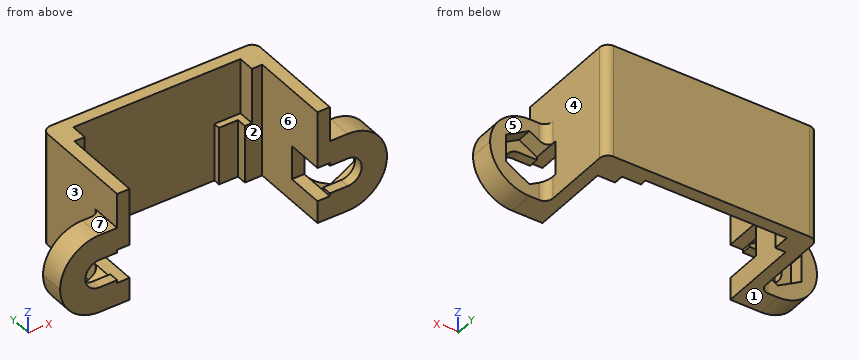
from build123d import *

# Parameters (mm, degrees)
BOSS_EXTRUDE1_DEPTH = 13.7
SKETCH3_W           = 6.9
SKETCH3_H           = 3
BOSS_EXTRUDE2_DEPTH = 9.5
SKETCH4_W           = 1.25
SKETCH4_H           = 2
BOSS_EXTRUDE3_DEPTH = 13.7
BOSS_EXTRUDE4_DEPTH = 7
CUT_EXTRUDE1_DEPTH  = 37.803396582
SKETCH7_W           = 2.15
SKETCH7_H           = 3.4
CUT_EXTRUDE2_DEPTH  = 37.803396582
CUT_EXTRUDE3_DEPTH  = 1.8
CUT_EXTRUDE4_REACH  = 38.457
SKETCH9_W           = 4.099186912
SKETCH9_H           = 4.5
FILLET1_R           = 1
FILLET2_R           = 1


with BuildPart() as part:
    # Sketch2 → Boss-Extrude1 (new body)
    with BuildSketch(Plane.XY):
        Polygon((0, 13.2), (0, 0), (1.5, 0), (1.5, 11.7), (24.2, 11.7), (24.2, 0), (25.7, 0), (25.7, 13.2), align=None)
    extrude(amount=BOSS_EXTRUDE1_DEPTH)

    # Sketch3 → Boss-Extrude2 (add)
    with BuildSketch(Plane(origin=(0, 0, 0), x_dir=(-1, 0, 0), z_dir=(0, 0, -1))):
        with Locations((-29.15, 1.5)):
            Rectangle(SKETCH3_W, SKETCH3_H)
        with Locations((3.45, 1.5)):
            Rectangle(SKETCH3_W, SKETCH3_H)
    extrude(amount=-BOSS_EXTRUDE2_DEPTH)

    # Sketch4 → Boss-Extrude3 (add)
    with BuildSketch(Plane(origin=(0, 0, 0), x_dir=(-1, 0, 0), z_dir=(0, 0, -1))):
        with Locations((-23.575, 10.7)):
            Rectangle(SKETCH4_W, SKETCH4_H)
        with Locations((-2.125, 10.7)):
            Rectangle(SKETCH4_W, SKETCH4_H)
    extrude(amount=-BOSS_EXTRUDE3_DEPTH)

    # Sketch5 → Boss-Extrude4 (add)
    with BuildSketch(Plane(origin=(0, 0, 0), x_dir=(-1, 0, 0), z_dir=(0, 0, -1))):
        Polygon((-22.95, 11.7), (-22.95, 9.7), (-22.1, 9.7), (-22.1, 10.9), (-19.8, 10.9), (-19.8, 11.7), align=None)
    extrude(amount=-BOSS_EXTRUDE4_DEPTH)

    # Sketch6 → Cut-Extrude1 (cut, through all)
    with BuildSketch(Plane(origin=(0, 3, 0), x_dir=(1, 0, 0), z_dir=(0, 1, 0))):
        with BuildLine():
            Line((32.6, -9.5), (32.6, -4.75))
            ThreePointArc((32.6, -4.75), (31.208757211, -8.108757211), (27.85, -9.5))
            Line((27.85, -9.5), (32.6, -9.5))
        make_face()
        with BuildLine():
            Line((32.6, -4.75), (32.6, 0))
            Line((32.6, 0), (27.85, 0))
            ThreePointArc((27.85, 0), (31.208757211, -1.391242789), (32.6, -4.75))
        make_face()
        with BuildLine():
            Line((-2.15, 0), (-6.9, 0))
            Line((-6.9, 0), (-6.9, -4.75))
            ThreePointArc((-6.9, -4.75), (-5.508757211, -1.391242789), (-2.15, 0))
        make_face()
        with BuildLine():
            ThreePointArc((-2.15, -9.5), (-5.508757211, -8.108757211), (-6.9, -4.75))
            Line((-6.9, -4.75), (-6.9, -9.5))
            Line((-6.9, -9.5), (-2.15, -9.5))
        make_face()
    extrude(amount=-CUT_EXTRUDE1_DEPTH, mode=Mode.SUBTRACT)

    # Sketch7 → Cut-Extrude2 (cut, through all)
    with BuildSketch(Plane(origin=(0, 3, 0), x_dir=(1, 0, 0), z_dir=(0, 1, 0))):
        with Locations((-1.075, -4.75)):
            Rectangle(SKETCH7_W, SKETCH7_H)
        with BuildLine():
            Line((-2.15, -6.45), (-2.15, -3.05))
            ThreePointArc((-2.15, -3.05), (-3.85, -4.75), (-2.15, -6.45))
        make_face()
    cut_extrude2 = extrude(amount=-CUT_EXTRUDE2_DEPTH, mode=Mode.SUBTRACT)

    # Sketch8 → Cut-Extrude3 (cut)
    with BuildSketch(Plane(origin=(0, 3, 0), x_dir=(1, 0, 0), z_dir=(0, 1, 0))):
        Polygon((-2.15, -8.040896534), (0.7, -6.395448267), (0.7, -3.104551733), (-2.15, -1.459103466), (-5, -3.104551733), (-5, -6.395448267), align=None)
        Polygon((30.7, -6.395448267), (27.85, -8.040896534), (25, -6.395448267), (25, -3.104551733), (27.85, -1.459103466), (30.7, -3.104551733), align=None)
    cut_extrude3 = extrude(amount=-CUT_EXTRUDE3_DEPTH, mode=Mode.SUBTRACT)

    # Cut-Extrude4: up to this face of the body (flat: up to its plane)
    cut_extrude4_end = Plane(part.part.faces().sort_by_distance((0, 7.554115794, 7.242871209))[0])
    # Sketch9 → Cut-Extrude4 (cut, up to the picked face)
    with BuildSketch(Plane(origin=(1.5, 0, 0), x_dir=(0, 0, -1), z_dir=(1, 0, 0)), mode=Mode.PRIVATE) as cut_extrude4_sk1:
        with Locations((-4.75, 2.25)):
            Rectangle(SKETCH9_W, SKETCH9_H)
    cut_extrude4_tool1 = split(extrude(cut_extrude4_sk1.sketch, amount=-CUT_EXTRUDE4_REACH, mode=Mode.PRIVATE), bisect_by=cut_extrude4_end, keep=Keep.BOTH, mode=Mode.PRIVATE)
    cut_extrude4 = cut_extrude4_tool1.solids().sort_by(Axis((1.5, 2.25, 4.75), (-1, 0, 0)))[0]
    add(cut_extrude4, mode=Mode.SUBTRACT)

    # Fillet1
    fillet1_edges = [part.edges().sort_by_distance(p)[0] for p in [
        (0, 3, 1.350203272),
        (25.7, 3, 1.350203272),
        (25.7, 3, 8.149796728),
        (0, 3, 8.149796728),
    ]]
    fillet(fillet1_edges, radius=FILLET1_R)

    # Mirror1: Cut-Extrude2, Cut-Extrude3, Cut-Extrude4 across plane
    add(cut_extrude2.mirror(Plane(origin=(12.85, 0, 0), x_dir=(0, 0, 1), z_dir=(1, 0, 0))), mode=Mode.SUBTRACT)
    add(cut_extrude3.mirror(Plane(origin=(12.85, 0, 0), x_dir=(0, 0, 1), z_dir=(1, 0, 0))), mode=Mode.SUBTRACT)
    add(cut_extrude4.mirror(Plane(origin=(12.85, 0, 0), x_dir=(0, 0, 1), z_dir=(1, 0, 0))), mode=Mode.SUBTRACT)

    # Fillet2
    fillet2_edges = [part.edges().sort_by_distance(p)[0] for p in [
        (0, 13.2, 6.85),
        (25.7, 13.2, 6.85),
    ]]
    fillet(fillet2_edges, radius=FILLET2_R)


solid = part.part
Can you work these out from the model? Positions are in its coordinate system, mm. Face numbers are marked on the shaded views. A direction names the side the tool comes from. Coordinates: 2 decimals unless noted, no trailing zeros. Loops run counter-clockwise (first coordinate to the right, second up) from the corner with the lowest first, then second, coordinate; pieces in that order, holes last. Notation, with made-up numbers: M 69.5,26.25 L 98.5,26.25 A19 cw 98.5,38.25 Z; hole C 80.5,53.25 d5. An arc over 180 degrees is marked long. Return JSON: item names as keys, results as strings. Group by question number.
Item 1: Imagine slicing it at D-D (y = 10.5). Please give me the cut outline in (x, z).
Item 2: On a 3-axis mill with a long thin cutter (end or side, diameter ignored), from which of +Z, -Z, +X, -X, +Y, -Y can I reach the whole of each face in a straight line? I mean the marked faces 4, 5, 6 and 7. Say none if no direction works.
Item 3: If I drill on L1, parallel to X at y = 11.5, z = 2.5; L2, parallel to X at y = 11, z = 10.75; L3, parallel to Z at x = 25.5, y = 1.75, over which ranges is the centre line in solid material (lowest first)? Write a range as from..to.
Item 4: Imagine slicing it at A-A (y = 6.5). Please give me the cut outline in (x, z), and give its area (3 significant figures).
Item 5: Imagine slicing it at C-C (x = 29). Please give me the cut outline in (y, z), and give its area (3 significant figures).
Item 6: Thinking about a two-plate mould opening in X: for the marked faces 1, 2 and 3, which applies, released by +X, released by -X, zero draft, split by the parting line, or undercut?
Item 7: Imagine slicing it at B-B (z = 5.5). Please give me the cut outline in (x, y).
Item 8: I'm going to push flat-ended pins straight in: pin 1 Ø1.3 at (x, y) = (-1.5, 1) entering from -Z; pin 2 Ø0.6 at (y, z) = (10.5, 5) entering from -X; pin 3 Ø3 at (x, z) = (29, 4) entering from +Y; pin 4 Ø1.6 at (x, z) = (0.5, 5) entering from -Y. Where does each tip first touch, or does it pass through?
Verdict:
{
 "1": {"outline": "M 0,0 L 2.75,0 L 2.75,13.7 L 0,13.7 Z; M 22.1,0 L 25.7,0 L 25.7,13.7 L 22.95,13.7 L 22.95,7 L 22.1,7 Z"},
 "2": {"face 4": "+Z, +X, +Y", "face 5": "+Z, -Z, +X, +Y", "face 6": "+Z, -Z, -Y", "face 7": "+Z, -X, +Y, -Y"},
 "3": {"L1": "x = 0..2.75, 19.8..25.7", "L2": "x = 0..2.75, 22.95..25.7", "L3": "z = 0..2.7, 6.8..13.7"},
 "4": {"outline": "M 0,0 L 1.5,0 L 1.5,13.7 L 0,13.7 Z; M 24.2,0 L 25.7,0 L 25.7,13.7 L 24.2,13.7 Z", "area": "41.1 mm^2"},
 "5": {"outline": "M 0,0.14 L 3,0.14 L 3,2.12 L 1.2,2.12 L 1.2,3.5 L 0,3.5 Z; M 0,6 L 1.2,6 L 1.2,7.38 L 3,7.38 L 3,9.36 L 0,9.36 Z", "area": "15.2 mm^2"},
 "6": {"face 1": "zero draft", "face 2": "undercut", "face 3": "released by -X"},
 "7": {"outline": "M -6.84,0 L -3.68,0 L -3.68,1.2 L -5,1.2 L -5,3 L -6.84,3 Z; M 0,4.5 L 1.5,4.5 L 1.5,9.7 L 2.75,9.7 L 2.75,11.7 L 19.8,11.7 L 19.8,10.9 L 22.1,10.9 L 22.1,9.7 L 24.2,9.7 L 24.2,4.5 L 25.7,4.5 L 25.7,12.2 A1 ccw 24.7,13.2 L 1,13.2 A1 ccw 0,12.2 Z; M 29.38,0 L 32.54,0 L 32.54,3 L 30.7,3 L 30.7,1.2 L 29.38,1.2 Z"},
 "8": {"pin 1": "stops at z = 0", "pin 2": "stops at x = 0", "pin 3": "stops at y = 1.2", "pin 4": "stops at y = 4.5"}
}
